Can you work these out from the model? Positions are in its coordinate system, mm. A direction names the side the tool comes from. Give positions to 0.01 mm unless a question says otherwise; leave off trailing zeros. Loops run counter-clockwise (first coordinate to the right, second up) from the corner with the lowest first, then second, coordinate; pieces in that order, holes last. Notation, with made-up numbers: (31, 37.5) - (57, 37.5) arc R14 ccw to (57, 62.5) - close; hole circle Ø7 at (38.25, 39.5). An arc over 180 degrees is marked (long way). Use a Markdown table: item, result. Add a question column.
```python
from build123d import *

# Parameters (mm, degrees)
SKETCH_1_W          = 15
SKETCH_1_H          = 15
SKETCH_1_W_2        = 12
SKETCH_1_H_2        = 12
EXTRUDE_1_DEPTH     = 460
SKETCH_2_R          = 2
CUT_EXTRUDE_1_DEPTH = 461.305605006
SKETCH_3_R          = 2
CUT_EXTRUDE_2_DEPTH = 461.305605006


with BuildPart() as part:
    # ｽｹｯﾁ1 → 押し出し-薄板1 (new body)
    with BuildSketch(Plane(origin=(0, 0, 0), x_dir=(1, 0, 0), z_dir=(0, 1, 0))):
        Rectangle(SKETCH_1_W, SKETCH_1_H)
        Rectangle(SKETCH_1_W_2, SKETCH_1_H_2, mode=Mode.SUBTRACT)
    extrude(amount=EXTRUDE_1_DEPTH)

    # ｽｹｯﾁ2 → ｶｯﾄ - 押し出し1 (cut, through all)
    with BuildSketch(Plane(origin=(7.5, 0, 0), x_dir=(0, 0, -1), z_dir=(1, 0, 0))):
        with Locations((0, 452.5)):
            Circle(SKETCH_2_R)
        with Locations((0, 427.5)):
            Circle(SKETCH_2_R)
    extrude(amount=-CUT_EXTRUDE_1_DEPTH, mode=Mode.SUBTRACT)

    # ｽｹｯﾁ3 → ｶｯﾄ - 押し出し2 (cut, through all)
    with BuildSketch(Plane.XY.offset(7.5)):
        with Locations((0, 7.5)):
            Circle(SKETCH_3_R)
        with Locations((0, 47.5)):
            Circle(SKETCH_3_R)
        with Locations((0, 27.5)):
            Circle(SKETCH_3_R)
        with Locations((0, 310)):
            Circle(SKETCH_3_R)
    extrude(amount=-CUT_EXTRUDE_2_DEPTH, mode=Mode.SUBTRACT)


solid = part.part
```
1. If we mould it in two halves opening along Z, with no side actions, what happens to faces 1 (the face through (0, 227, 6)), 2 (the face through (-6, 227, 0)), 3 (the face through (-7.5, 227, 0)), 4 (the face through (0, 227, 7.5))? For each: released by +Z, released by -Z, zero draft, split by the parting line, or undercut.
2. Suppose I cut it at A-A (y = 349). List the corners of the cut face in (x, z) for me, and give its area (3 significant figures).
3. On a 3-axis mill with a long thin cutter (end or side, diameter ignored), from which of +Z, -Z, +X, -X, +Y, -Y can I reach the whole of each face in a straight line? I mean faces 5 (the face through (-7, 460, 0)), 6 (the face through (6, 227, 0)). Say none if no direction works.
4. Please list where these lines run through material, in increasing order: line 1 along Y through (x, z) = (0, -6.35); line 2 along Z through (x, y) = (0.25, 225.5); line 3 along Y through (x, z) = (6.85, 0). Write a range as [from, to].
Results below:
| question | item | result |
|---|---|---|
| 1 | face 1 | undercut |
| 1 | face 2 | undercut |
| 1 | face 3 | zero draft |
| 1 | face 4 | released by +Z |
| 2 | outline | (-7.5, -7.5) - (7.5, -7.5) - (7.5, 7.5) - (-7.5, 7.5) - close; hole (-6, -6) - (6, -6) - (6, 6) - (-6, 6) - close |
| 2 | area | 81.0 mm² |
| 3 | face 5 | +Z, -Z, +X, -X, +Y |
| 3 | face 6 | +Y, -Y |
| 4 | line 1 | [0, 5.5], [9.5, 25.5], [29.5, 45.5], [49.5, 308], [312, 460] |
| 4 | line 2 | [-7.5, -6], [6, 7.5] |
| 4 | line 3 | [0, 425.5], [429.5, 450.5], [454.5, 460] |
